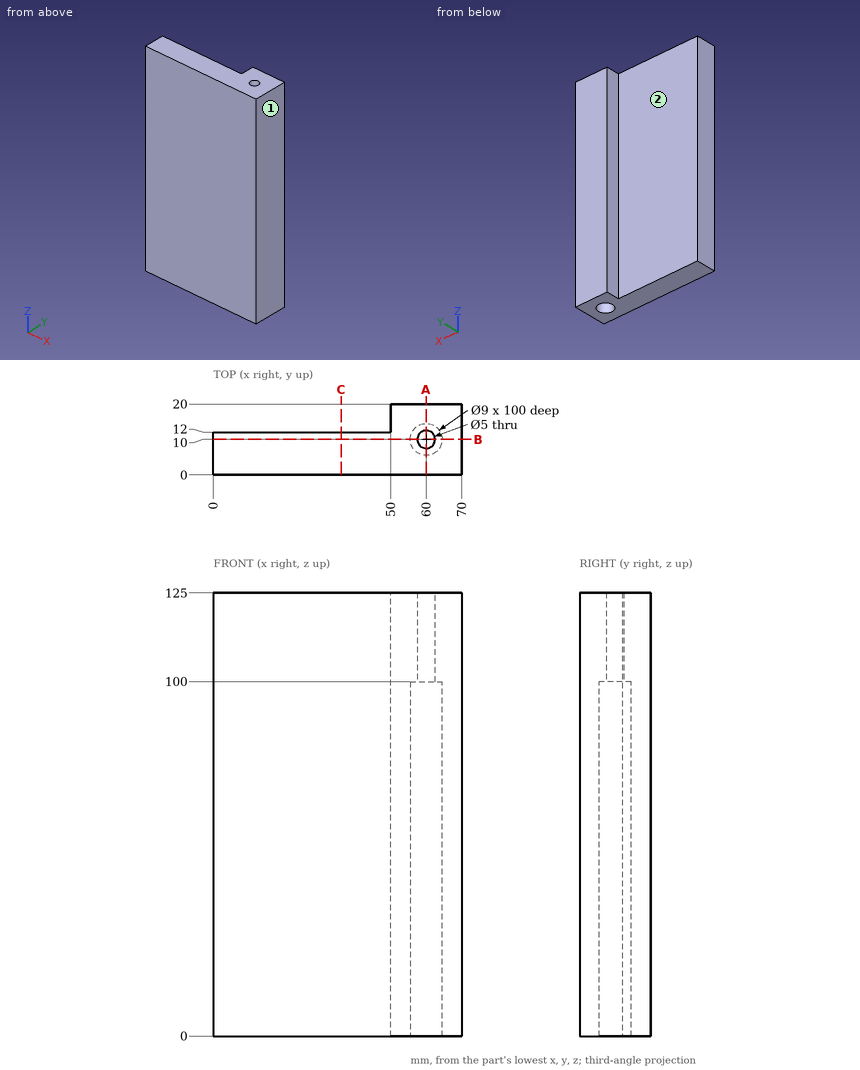
For this review, use the dimensioned drawing (mm, ordinates from the lowest corner) and the shaded views. A direction names the side the tool comes from. Give positions to 0.01 mm unless a question says otherwise; leave off trailing zeros. Order: outer loops, then holes, each group sorted by start corner. A loop starts at its lowest first (then second) coordinate and runs counter-clockwise, first axis right, second up. Notation, with made-up numbers: M -21,-35.75 L 17,-35.75 A13 cw 17,-10.75 Z; hole C -25.75,64 d6. An arc over 180 degrees is marked long. Use one line per item in the form item = value. Start each with the question number.
Item 1: For the marked faces 1 and 2, list the 3-axis set-ups (+Z, -Z, +X, -X, +Y, -Y) from which the entire face can be reached by the end or side of a thin tool; tool diameter is ignored.
Item 2: We need section C-C on x = 36. Give the boundary of the cut face in (y, z).
Item 3: We need section A-A on x = 60. Give the boundary of the cut face in (y, z).
Item 4: To check wall thickness, follow line 1 along Y through (x, z) = (60, 116); line 2 along Y through (x, z) = (60, 42); line 3 along Y through (x, z) = (24, 8). State the ranges of each line that lie inside material, in increasing order. Write a range as from..to.
Item 5: We need section B-B on y = 10. Give the boundary of the cut face in (x, z), plus the area to 4 significant figures.
Item 6: Insertion check: pin 1 Ø2.5 at (y, z) = (16, 59.5) entering from -X; pin 2 Ø1.5 at (x, z) = (30, 73) entering from +Y. Each pin has a flat end and moves straight along its axis. Give the tip position at first contact, or say it passes through.
Completed:
q1.face_1 = +Z, -Z, +X, +Y, -Y
q1.face_2 = +Z, -Z, -X, +Y
q2.outline = M 0,0 L 12,0 L 12,125 L 0,125 Z
q3.outline = M 0,0 L 5.5,0 L 5.5,100 L 7.5,100 L 7.5,125 L 0,125 Z; M 12.5,100 L 14.5,100 L 14.5,0 L 20,0 L 20,125 L 12.5,125 Z
q4.line_1 = 0..7.5, 12.5..20
q4.line_2 = 0..5.5, 14.5..20
q4.line_3 = 0..12
q5.outline = M 0,0 L 55.5,0 L 55.5,100 L 57.5,100 L 57.5,125 L 0,125 Z; M 62.5,100 L 64.5,100 L 64.5,0 L 70,0 L 70,125 L 62.5,125 Z
q5.area = 7,725 mm²
q6.pin_1 = 50
q6.pin_2 = 12
